Work out the finished part from the listing and answer in its coordinate system (mm). Face numbers are marked on the shaded views. Round coordinates to 2 decimals unless told otherwise and drop trailing zeros. Write each loop counter-clockwise with the first axis right and the second up, starting at its lowest first coordinate (ties: lowest second). Pieces come first, ordered by that corner, then holes. Notation, with made-up numbers: (-15, -6) -> (0, -6) arc R15 cw to (0, 23) -> close; hole circle Ø6 at (72.5, 16). An arc over 180 degrees is marked (long way). Answer as a JSON object with one key per item and string values. Group by question number.
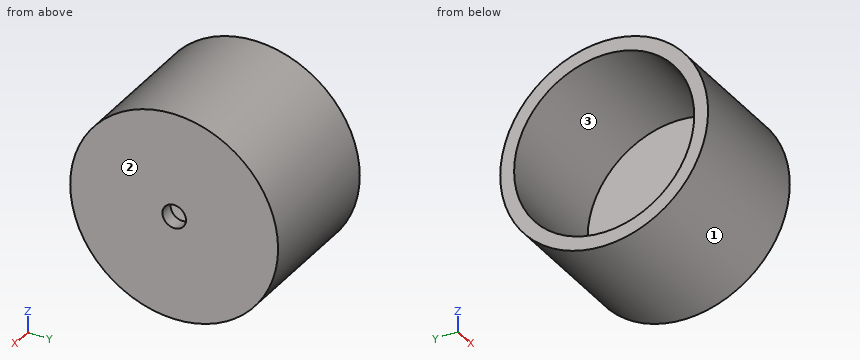
from build123d import *

# Parameters (mm, degrees)
SKETCH1_R           = 15
BOSS_EXTRUDE3_DEPTH = 20
SHELL2_T            = -2
SKETCH2_R           = 1.7
CUT_EXTRUDE1_DEPTH  = 2


with BuildPart() as part:
    # Sketch1 → Boss-Extrude3 (new body)
    with BuildSketch(Plane(origin=(0, 0, 0), x_dir=(0, 0, -1), z_dir=(1, 0, 0))):
        Circle(SKETCH1_R)
    extrude(amount=BOSS_EXTRUDE3_DEPTH)

    # Shell2
    shell2_openings = [part.faces().sort_by_distance(p)[0] for p in [
        (0, 0, 0),
    ]]
    offset(amount=SHELL2_T, openings=shell2_openings, kind=Kind.INTERSECTION)

    # Sketch2 → Cut-Extrude1 (cut)
    with BuildSketch(Plane(origin=(20, 0, 0), x_dir=(0, 0, -1), z_dir=(1, 0, 0))):
        Circle(SKETCH2_R)
    extrude(amount=-CUT_EXTRUDE1_DEPTH, mode=Mode.SUBTRACT)


solid = part.part
1) For a pull along Y with two mould halves and no side action, classify the marked faces 1, 2 and 3 as released by +Y, released by -Y, zero draft, split by the parting line, or undercut.
2) A cutting plane is placed at A-A on z = 0. Determine the outline of the cut face in (x, y).
3) Straight lines are drawn through the part: L1, parallel to Y at x = 19.5, z = 0; L2, parallel to X at y = 10.5, z = 2; L3, parallel to Y at x = 6, z = 0. For each, find the intervals that lie inside material, in ascending order.
4) A cutting plane is placed at D-D on z = 3.5. Determine the outline of the cut face in (x, y), plus the area to 3 significant figures.
5) A cutting plane is placed at C-C on x = 9.5. Determine the outline of the cut face in (y, z).
6) Each of these flat-tipped pins is pushed along its axis until it touches: P1, Ø15.5, axis at y = 0, z = 0, coming from the +X side; P2, Ø1, axis at y = 6, z = 9, coming from the -X side; P3, Ø1, axis at x = 5, z = 7, coming from the +Y side; P4, Ø5, axis at x = 5, y = -11.5, coming from the +Z side. Where does it stop, or does it pass through?
Established:
{
 "1": {"face 1": "split by the parting line", "face 2": "zero draft", "face 3": "undercut"},
 "2": {"outline": "(0, -15) -> (20, -15) -> (20, -1.7) -> (18, -1.7) -> (18, -13) -> (0, -13) -> close; (0, 13) -> (18, 13) -> (18, 1.7) -> (20, 1.7) -> (20, 15) -> (0, 15) -> close"},
 "3": {"L1": "y = -15 to -1.7, 1.7 to 15", "L2": "x = 18 to 20", "L3": "y = -15 to -13, 13 to 15"},
 "4": {"outline": "(0, -14.59) -> (20, -14.59) -> (20, 14.59) -> (0, 14.59) -> (0, 12.52) -> (18, 12.52) -> (18, -12.52) -> (0, -12.52) -> close", "area": "133 mm²"},
 "5": {"outline": "circle Ø30 at (0, 0); hole circle Ø26 at (0, 0)"},
 "6": {"P1": "stops at x = 20", "P2": "stops at x = 18", "P3": "stops at y = 13.52", "P4": "stops at z = 12"}
}
